Read the model definition and answer for the solid it produces. Units are mm, in the model's axes. A direction names the side the tool comes from. Give positions to 0.01 mm unless a question says otherwise; leave off trailing zeros. Loops run counter-clockwise (first coordinate to the right, second up) from the corner with the lowest first, then second, coordinate; pieces in that order, holes last. Notation, with made-up numbers: (24.5, 25.25) - (73.5, 25.25) arc R32 ccw to (73.5, 57.25) - close; hole circle Ø3 at (86, 26). An arc over 180 degrees is marked (long way). Use a Markdown table: item, result. Add a question column.
Item 1: A cutting plane is placed at B-B (x = 109). Determine the outline of the cut face in (y, z), plus the area to 4 significant figures.
Item 2: Consider probe 1 along Z at (x, y) = (280, 27); probe 2 along Y at (x, z) = (-14, -21); probe 3 along Y at (x, z) = (-39, 2.5). Determine where each line is inside the solid, lowest interval first. Write a range as [from, to].
Item 3: A cutting plane is placed at A-A (y = 18). Determine the outline of the cut face in (x, z), plus the area to 3 significant figures.
Item 4: Which of the six approach directions +Z, -Z, +X, -X, +Y, -Y give full straight-line access (tool end or side, diameter ignored) to faces 1 (the face through (16, 2.5, -8)), 2 (the face through (16, 30, -26))?
Item 5: A cutting plane is placed at C-C (z = -12). Determine the outline of the cut face in (x, y).
from build123d import *

# Parameters (mm, degrees)
SKETCH1_W           = 600
SKETCH1_H           = 50
BOSS_EXTRUDE1_DEPTH = 30
SKETCH2_W           = 40
SKETCH2_H           = 25
CUT_EXTRUDE1_DEPTH  = 602.62290577
SKETCH3_W           = 600
SKETCH3_H           = 25
CUT_EXTRUDE2_DEPTH  = 20


with BuildPart() as part:
    # Sketch1 → Boss-Extrude1 (new body)
    with BuildSketch(Plane(origin=(0, 0, 0), x_dir=(1, 0, 0), z_dir=(0, 1, 0))):
        with Locations((20.477137177, 7.4055666)):
            Rectangle(SKETCH1_W, SKETCH1_H)
    extrude(amount=BOSS_EXTRUDE1_DEPTH)

    # Sketch2 → Cut-Extrude1 (cut, through all)
    with BuildSketch(Plane.ZY.offset(279.522862823)):
        with Locations((-7.4055666, 15)):
            Rectangle(SKETCH2_W, SKETCH2_H)
    extrude(amount=-CUT_EXTRUDE1_DEPTH, mode=Mode.SUBTRACT)

    # Sketch3 → Cut-Extrude2 (cut)
    with BuildSketch(Plane(origin=(0, 30, 0), x_dir=(1, 0, 0), z_dir=(0, 1, 0))):
        with Locations((20.477137177, 7.4055666)):
            Rectangle(SKETCH3_W, SKETCH3_H)
    extrude(amount=-CUT_EXTRUDE2_DEPTH, mode=Mode.SUBTRACT)


solid = part.part
Geometry says:
| question | item | result |
|---|---|---|
| 1 | outline | (0, -32.41) - (30, -32.41) - (30, -19.91) - (27.5, -19.91) - (27.5, -27.41) - (2.5, -27.41) - (2.5, 12.59) - (27.5, 12.59) - (27.5, 5.09) - (30, 5.09) - (30, 17.59) - (0, 17.59) - close |
| 1 | area | 437.5 mm² |
| 2 | probe 1 | [-32.41, -27.41], [12.59, 17.59] |
| 2 | probe 2 | [0, 2.5], [27.5, 30] |
| 2 | probe 3 | [0, 2.5] |
| 3 | outline | (-279.52, -32.41) - (320.48, -32.41) - (320.48, -27.41) - (-279.52, -27.41) - close; (-279.52, 12.59) - (320.48, 12.59) - (320.48, 17.59) - (-279.52, 17.59) - close |
| 3 | area | 6,000 mm² |
| 4 | face 1 | +X, -X |
| 4 | face 2 | +Z, -Z, +X, -X, +Y |
| 5 | outline | (-279.52, 0) - (320.48, 0) - (320.48, 2.5) - (-279.52, 2.5) - close |
